Read the model definition and answer for the solid it produces. Units are mm, in the model's axes. A direction names the side the tool comes from. Round coordinates to 2 decimals unless told otherwise and drop trailing zeros. Write each loop counter-clockwise with the first axis right and the second up, starting at its lowest first coordinate (ties: lowest second). Pieces come first, ordered by that corner, then holes. Notation, with made-up numbers: (56.25, 1.25) - (86.25, 1.25) arc R21 cw to (86.25, 20.25) - close; hole circle Ø2 at (3.5, -38.75). An arc over 180 degrees is marked (long way). Use one line per item in the form item = value. Start each with the question number.
1) The part is cut by section C-C, the plane y = -97.5. Give the vertices of the cut face in (x, z).
2) The part is cut by section B-B, the plane z = -406.4. Give the vertices of the cut face in (x, y), plus the area to 3 significant figures.
3) For faces 1 (the face through (330.2, -225, -5)), 2 (the face through (-269, -406.4, -406)), 3 (the face through (-269, -368.3, -406)), determine the directions among +Z, -Z, +X, -X, +Y, -Y from which every point of the face is accessible in a straight line to the end or side of a thin tool.
4) The part is cut by section A-A, the plane x = -266.7. Give the vertices of the cut face in (y, z).
5) Consider line 1 along Z through (x, y) = (-35, -98.5); line 2 along Z through (x, y) = (-279, -404.5). Determine where each line is inside the solid, lowest interval first. Write a range as from..to.
6) For a pull along Z with two mould halves and no side action, classify faces 4 (the face through (-5, -225, 374.65)), 5 (the face through (-267.66, -387.617, -438.135)), 6 (the face through (-5, 0, 5)) as released by +Z, released by -Z, zero draft, split by the parting line, or undercut.
from build123d import *

# Parameters (mm, degrees)
F0_W     = 660.4
F0_H     = 749.3
F1_DEPTH = 457.2
F4_DEPTH = 38.1


with BuildPart() as f1:
    # F0 (on Front) → F1 (new body)
    with BuildSketch(Plane.XZ):
        Rectangle(F0_W, F0_H)
    extrude(amount=F1_DEPTH)

    # F3 (on offset) → F4 (join)
    with BuildSketch(Plane.XZ.offset(406.4)):
        with BuildLine():
            Line((-301.641643, -374.65), (-293.075598, -388.725433))
            ThreePointArc((-293.075598, -388.725433), (-266.7, -438.15), (-240.324402, -388.725433))
            Line((-240.324402, -388.725433), (-235.105276, -374.65))
            Line((-235.105276, -374.65), (-301.641643, -374.65))
        make_face()
    extrude(amount=-F4_DEPTH)


solid = f1.part
Geometry results:
q1.outline = (-330.2, -374.65) - (330.2, -374.65) - (330.2, 374.65) - (-330.2, 374.65) - close
q2.outline = (-298.45, -406.4) - (-234.95, -406.4) - (-234.95, -368.3) - (-298.45, -368.3) - close
q2.area = 2,420 mm2
q3.face_1 = +Z, -Z, +X, +Y, -Y
q3.face_2 = -Z, +X, -X, -Y
q3.face_3 = -Z, +X, -X, +Y
q4.outline = (-457.2, -374.65) - (-406.4, -374.65) - (-406.4, -438.15) - (-368.3, -438.15) - (-368.3, -374.65) - (0, -374.65) - (0, 374.65) - (-457.2, 374.65) - close
q5.line_1 = -374.65..374.65
q5.line_2 = -435.67..374.65
q6.face_4 = released by +Z
q6.face_5 = undercut
q6.face_6 = zero draft
